```python
from build123d import *

# Parameters (mm, degrees)
PAD_DEPTH       = 51
PAD001_DEPTH    = 22
PAD002_DEPTH    = 66
PAD003_DEPTH    = 1
PAD004_DEPTH    = 25
PAD005_DEPTH    = 51
PAD006_DEPTH    = 17
PAD007_DEPTH    = 17
PAD008_DEPTH    = 17
PAD009_DEPTH    = 41
SKETCH010_W     = 2
SKETCH010_H     = 1
PAD010_DEPTH    = 7
POCKET_DEPTH    = 1
PAD011_DEPTH    = 68
POCKET001_DEPTH = 68
POCKET002_DEPTH = 70
POCKET003_DEPTH = 22
POCKET004_DEPTH = 54
POCKET005_DEPTH = 17
SKETCH018_W     = 3
SKETCH018_H     = 2
POCKET006_DEPTH = 2
POCKET007_DEPTH = 17
PAD012_DEPTH    = 17
PAD013_DEPTH    = 18
POCKET008_DEPTH = 70
SKETCH023_W     = 3
SKETCH023_H     = 5
PAD014_DEPTH    = 103
POCKET009_DEPTH = 13
SKETCH025_W     = 2
SKETCH025_H     = 3
POCKET010_DEPTH = 103
SKETCH026_W     = 3
SKETCH026_H     = 5
PAD015_DEPTH    = 103
SKETCH027_W     = 2
SKETCH027_H     = 3
POCKET011_DEPTH = 103
POCKET012_DEPTH = 31
POCKET013_DEPTH = 45
POCKET014_DEPTH = 28
PAD016_DEPTH    = 44
POCKET015_DEPTH = 51
SKETCH033_W     = 6
SKETCH033_H     = 7
POCKET016_DEPTH = 2


with BuildPart() as part:
    # Sketch → Pad (new body)
    with BuildSketch(Plane.XZ):
        Polygon((0, 0), (15, 0), (15, -2), (14, -3), (1, -3), (0, -2), align=None)
    extrude(amount=PAD_DEPTH)

    # Sketch001 (on Face2 of Pad) → Pad001 (join)
    with BuildSketch(Plane(origin=(5, 0, 0), x_dir=(0, 0, 1), z_dir=(1, 0, 0))):
        Polygon((0, 51), (0, 66), (-2, 66), (-3, 65), (-3, 52), (-2, 51), align=None)
    extrude(amount=PAD001_DEPTH)

    # Sketch002 (on Face14 of Pad001) → Pad002 (join)
    with BuildSketch(Plane(origin=(27, 0, 0), x_dir=(0, 0, 1), z_dir=(1, 0, 0))):
        Polygon((0, 70), (0, 55), (-2, 55), (-3, 56), (-3, 69), (-2, 70), align=None)
    extrude(amount=PAD002_DEPTH)

    # Sketch004 (on Face5 of Pad002) → Pad003 (join)
    with BuildSketch(Plane.XZ.offset(51)):
        Polygon((0, 0), (15, 0), (15, -2), (14, -3), (1, -3), (0, -2), align=None)
    extrude(amount=PAD003_DEPTH)

    # Sketch003 (on Face20 of Pad002) → Pad004 (join)
    with BuildSketch(Plane(origin=(0, -56, 0), x_dir=(1, 0, 0), z_dir=(0, 1, 0))):
        Polygon((93, 0), (78, 0), (78, 2), (79, 3), (92, 3), (93, 2), align=None)
    extrude(amount=PAD004_DEPTH)

    # Sketch005 (on Face38 of Pad004) → Pad005 (join)
    with BuildSketch(Plane(origin=(0, -31, 0), x_dir=(1, 0, 0), z_dir=(0, 1, 0))):
        Polygon((84, 0), (99, 0), (99, 2), (98, 3), (85, 3), (84, 2), align=None)
    extrude(amount=PAD005_DEPTH)

    # Sketch006 (on Face47 of Pad005) → Pad006 (join)
    with BuildSketch(Plane(origin=(0, 13, 0), x_dir=(1, 0, 0), z_dir=(0, 1, 0))):
        Polygon((69, 0), (84, 0), (84, 2), (83, 3), (70, 3), (69, 2), align=None)
    extrude(amount=PAD006_DEPTH)

    # Sketch007 (on Face4 of Pad006) → Pad007 (join)
    with BuildSketch(Plane(origin=(0, 0, 0), x_dir=(1, 0, 0), z_dir=(0, 1, 0))):
        Polygon((8, 0), (23, 0), (23, 2), (22, 3), (9, 3), (8, 2), align=None)
    extrude(amount=PAD007_DEPTH)

    # Sketch008 (on Face17 of Pad007) → Pad008 (join)
    with BuildSketch(Plane(origin=(0, 17, 0), x_dir=(1, 0, 0), z_dir=(0, 1, 0))):
        Polygon((15, 0), (30, 0), (30, 2), (29, 3), (16, 3), (15, 2), align=None)
    extrude(amount=PAD008_DEPTH)

    # Sketch009 (on Face31 of Pad008) → Pad009 (join)
    with BuildSketch(Plane(origin=(29, 0, 0), x_dir=(0, 0, 1), z_dir=(1, 0, 0))):
        Polygon((0, -37), (0, -22), (-2, -22), (-3, -23), (-3, -36), (-2, -37), align=None)
    extrude(amount=PAD009_DEPTH)

    # Sketch010 (on Face81 of Pad009) → Pad010 (join)
    with BuildSketch(Plane(origin=(0, 13, 0), x_dir=(1, 0, 0), z_dir=(0, 1, 0))):
        with Locations((84, 2.5)):
            Rectangle(SKETCH010_W, SKETCH010_H)
    extrude(amount=PAD010_DEPTH)

    # Sketch011 (on Face36 of Pad010) → Pocket (cut)
    with BuildSketch(Plane(origin=(0, 0, 0), x_dir=(-1, 0, 0), z_dir=(0, 0, 1))):
        Polygon((-90.1471723822, 70), (-79, 70), (-90.1471723822, 59.9630409046), align=None)
    extrude(amount=-POCKET_DEPTH, mode=Mode.SUBTRACT)

    # Sketch012 (on Face51 of Pocket) → Pad011 (join)
    with BuildSketch(Plane(origin=(38.0611229336, -42.2711594585, 0), x_dir=(0.7431448255, 0.6691306064, 0), z_dir=(0.6691306064, -0.7431448255, 0))):
        Polygon((11.8692987676, 0), (26.8692987676, 0), (26.8692987676, -2), (25.8692987676, -3), (12.8692987676, -3), (11.8692987676, -2), align=None)
    extrude(amount=PAD011_DEPTH)

    # Sketch013 (on Face80 of Pad011) → Pocket001 (cut)
    with BuildSketch(Plane(origin=(83.562004166, -92.805007591, 0), x_dir=(0.7431448255, 0.6691306064, 0), z_dir=(0.6691306064, -0.7431448255, 0))):
        Polygon((14.8692987676, 0), (23.8692987676, 0), (23.8692987676, -1.5), (24.3692987676, -1.5), (24.3692987676, -2), (14.3692987676, -2), (14.3692987676, -1.5), (14.8692987676, -1.5), align=None)
    extrude(amount=-POCKET001_DEPTH, mode=Mode.SUBTRACT)

    # Sketch014 (on Face46 of Pocket001) → Pocket002 (cut)
    with BuildSketch(Plane(origin=(27, 0, 0), x_dir=(0, 0, -1), z_dir=(-1, 0, 0))):
        Polygon((0, 67), (1.5, 67), (1.5, 67.5), (2, 67.5), (2, 57.5), (1.5, 57.5), (1.5, 58), (0, 58), align=None)
    extrude(amount=-POCKET002_DEPTH, mode=Mode.SUBTRACT)

    # Sketch015 (on Face34 of Pocket002) → Pocket003 (cut)
    with BuildSketch(Plane(origin=(5, 0, 0), x_dir=(0, 0, -1), z_dir=(-1, 0, 0))):
        Polygon((0, 63), (0.5, 63), (0.5, 63.5), (2, 63.5), (2, 53.5), (0.5, 53.5), (0.5, 54), (0, 54), align=None)
    extrude(amount=-POCKET003_DEPTH, mode=Mode.SUBTRACT)

    # Sketch016 (on Face4 of Pocket003) → Pocket004 (cut)
    with BuildSketch(Plane(origin=(0, 0, 0), x_dir=(1, 0, 0), z_dir=(0, 1, 0))):
        Polygon((2.5, 2), (12.5, 2), (12.5, 1.5), (12, 1.5), (12, 0), (3, 0), (3, 1.5), (2.5, 1.5), align=None)
    extrude(amount=-POCKET004_DEPTH, mode=Mode.SUBTRACT)

    # Sketch017 (on Face19 of Pocket004) → Pocket005 (cut)
    with BuildSketch(Plane(origin=(0, 17, 0), x_dir=(1, 0, 0), z_dir=(0, 1, 0))):
        Polygon((11, 0), (11, 1.5), (10.5, 1.5), (10.5, 2), (20.5, 2), (20.5, 1.5), (20, 1.5), (20, 0), align=None)
    extrude(amount=-POCKET005_DEPTH, mode=Mode.SUBTRACT)

    # Sketch018 (on Face48 of Pocket005) → Pocket006 (cut)
    with BuildSketch(Plane(origin=(0, 0, 0), x_dir=(-1, 0, 0), z_dir=(0, 0, 1))):
        with Locations((-11.5, 0)):
            Rectangle(SKETCH018_W, SKETCH018_H)
    extrude(amount=-POCKET006_DEPTH, mode=Mode.SUBTRACT)

    # Sketch019 (on Face63 of Pocket006) → Pocket007 (cut)
    with BuildSketch(Plane(origin=(0, 34, 0), x_dir=(1, 0, 0), z_dir=(0, 1, 0))):
        Polygon((18, 0), (18, 1.5), (17.5, 1.5), (17.5, 2), (27.5, 2), (27.5, 1.5), (27, 1.5), (27, 0), align=None)
    extrude(amount=-POCKET007_DEPTH, mode=Mode.SUBTRACT)

    # Sketch020 (on Face117 of Pocket007) → Pad012 (join)
    with BuildSketch(Plane(origin=(0, 30, 0), x_dir=(1, 0, 0), z_dir=(0, 1, 0))):
        Polygon((70, 3), (83, 3), (84, 2), (84, 0), (69, 0), (69, 2), align=None)
    extrude(amount=PAD012_DEPTH)

    # Sketch021 (on Face108 of Pad012) → Pad013 (join)
    with BuildSketch(Plane.XZ.offset(74.8)):
        Polygon((88.5297845093, 0), (103.5297845093, 0), (103.5297845093, -2), (102.5297845093, -3), (89.5297845093, -3), (88.5297845093, -2), align=None)
    extrude(amount=PAD013_DEPTH)

    # Sketch022 (on Face158 of Pad013) → Pocket008 (cut)
    with BuildSketch(Plane(origin=(38.0611229336, -42.2711594585, 0), x_dir=(0.7431448255, 0.6691306064, 0), z_dir=(-0.6691306064, 0.7431448255, 0))):
        Polygon((14.3692987676, 2), (24.3692987676, 2), (24.3692987676, 1.5), (23.8692987676, 1.5), (23.8692987676, 0), (14.8692987676, 0), (14.8692987676, 1.5), (14.3692987676, 1.5), align=None)
    extrude(amount=-POCKET008_DEPTH, mode=Mode.SUBTRACT)

    # Sketch023 (on Face171 of Pocket008) → Pad014 (join)
    with BuildSketch(Plane(origin=(103.5297845093, 0, 0), x_dir=(0, 0, -1), z_dir=(-1, 0, 0))):
        with Locations((1.5, 90.3)):
            Rectangle(SKETCH023_W, SKETCH023_H)
    extrude(amount=PAD014_DEPTH)

    # Sketch024 (on Face231 of Pad014) → Pocket009 (cut)
    with BuildSketch(Plane.XZ.offset(92.8)):
        Polygon((91.0297845093, -2), (101.0297845093, -2), (101.0297845093, -1.5), (100.5297845093, -1.5), (100.5297845093, 0), (91.5297845093, 0), (91.5297845093, -1.5), (91.0297845093, -1.5), align=None)
    extrude(amount=-POCKET009_DEPTH, mode=Mode.SUBTRACT)

    # Sketch025 (on Face210 of Pocket009) → Pocket010 (cut)
    with BuildSketch(Plane(origin=(0.5297845093, 0, 0), x_dir=(0, 0, -1), z_dir=(-1, 0, 0))):
        with Locations((1, 91.3)):
            Rectangle(SKETCH025_W, SKETCH025_H)
    extrude(amount=-POCKET010_DEPTH, mode=Mode.SUBTRACT)

    # Sketch026 (on Face150 of Pocket010) → Pad015 (join)
    with BuildSketch(Plane(origin=(0.5, 0, 0), x_dir=(0, 0, 1), z_dir=(1, 0, 0))):
        with Locations((-1.5, -44.5)):
            Rectangle(SKETCH026_W, SKETCH026_H)
    extrude(amount=PAD015_DEPTH)

    # Sketch027 (on Face187 of Pad015) → Pocket011 (cut)
    with BuildSketch(Plane(origin=(103.5, 0, 0), x_dir=(0, 0, 1), z_dir=(1, 0, 0))):
        with Locations((-1, -45.5)):
            Rectangle(SKETCH027_W, SKETCH027_H)
    extrude(amount=-POCKET011_DEPTH, mode=Mode.SUBTRACT)

    # Sketch028 (on Face117 of Pocket011) → Pocket012 (cut)
    with BuildSketch(Plane.XZ.offset(-13)):
        Polygon((71.5, -2), (81.5, -2), (81.5, -1.5), (81, -1.5), (81, 0), (72, 0), (72, -1.5), (71.5, -1.5), align=None)
    extrude(amount=-POCKET012_DEPTH, mode=Mode.SUBTRACT)

    # Sketch029 (on Face87 of Pocket012) → Pocket013 (cut)
    with BuildSketch(Plane(origin=(27, 0, 0), x_dir=(0, 0, -1), z_dir=(-1, 0, 0))):
        Polygon((2, -24.5), (2, -34.5), (1.5, -34.5), (1.5, -34), (0, -34), (0, -25), (1.5, -25), (1.5, -24.5), align=None)
    extrude(amount=-POCKET013_DEPTH, mode=Mode.SUBTRACT)

    # Sketch030 (on Face210 of Pocket013) → Pocket014 (cut)
    with BuildSketch(Plane(origin=(0, -31, 0), x_dir=(1, 0, 0), z_dir=(0, 1, 0))):
        Polygon((80.5, 2), (90.5, 2), (90.5, 1.5), (90, 1.5), (90, 0), (81, 0), (81, 1.5), (80.5, 1.5), align=None)
    extrude(amount=-POCKET014_DEPTH, mode=Mode.SUBTRACT)

    # Sketch031 (on Face234 of Pocket014) → Pad016 (join)
    with BuildSketch(Plane(origin=(0, -31, 0), x_dir=(1, 0, 0), z_dir=(0, 1, 0))):
        Polygon((78, 2), (79, 3), (85, 3), (85, 2), (80.5, 2), (80.5, 1.5), (81, 1.5), (81, 0), (78, 0), align=None)
    extrude(amount=PAD016_DEPTH)

    # Sketch032 (on Face205 of Pad016) → Pocket015 (cut)
    with BuildSketch(Plane(origin=(0, 20, 0), x_dir=(1, 0, 0), z_dir=(0, 1, 0))):
        Polygon((86.5, 2), (96.5, 2), (96.5, 1.5), (96, 1.5), (96, 0), (87, 0), (87, 1.5), (86.5, 1.5), align=None)
    extrude(amount=-POCKET015_DEPTH, mode=Mode.SUBTRACT)

    # Sketch033 (on Face207 of Pocket015) → Pocket016 (cut)
    with BuildSketch(Plane(origin=(0, 0, 0), x_dir=(-1, 0, 0), z_dir=(0, 0, 1))):
        with Locations((-84, -16.5)):
            Rectangle(SKETCH033_W, SKETCH033_H)
    extrude(amount=-POCKET016_DEPTH, mode=Mode.SUBTRACT)


solid = part.part
```
For this review, take the finished solid that the model builds, in its own axes (mm). A direction names the side the tool comes from. Round coordinates to 2 decimals unless told otherwise and drop trailing zeros. Write each loop counter-clockwise with the first axis right and the second up, starting at its lowest first coordinate (ties: lowest second). Pieces come first, ordered by that corner, then holes. Notation, with made-up numbers: M 23.25,-25.75 L 46.25,-25.75 A22 ccw 46.25,7.25 Z; hole C 82.25,26.5 d7. An arc over 180 degrees is marked long. One line per item, written item: value. Start each with the question number.
(1) Machinability: for faces 1 (the flat face through (43.7, 42.4, 0)), 2 (the flat face through (20.3, 34, -2.2)), 3 (the flat face through (98.224, -72.669, -1.754)), 4 (the flat face through (67.875, -35.227, -0.986)), which of the approach directions +Z, -Z, +X, -X, +Y, -Y give a long, thin tool a straight path to every point of the face, cutting with its end or side? Answer none if there is none.
(2) Insertion check: pin 1 (1.2 mm diameter, centred on y = -14.5, z = -1, fed in from +X); pin 2 (0.8 mm diameter, centred on y = 9, z = -0.5, fed in from -X); pin 3 (0.9 mm diameter, centred on y = -44, z = -2, fed in from +X); pin 4 (10 mm diameter, centred on x = 50.5, y = -18, fed in from +Z). Each pin has a flat end and moves straight along its axis. Give the tip position at first contact, or say it passes through.
(3) We need section C-C (x = 42). Count the separate pieces of the cut face and the enclosed holes in it, and give its area (3 significant figures).
(4) Wall thickness on line 1 (X direction, y = -21.5, z = -1.8); line 2 (Y direction, x = 17, z = -1); line 3 (X direction, y = -10.5, z = -0.3): over which ranges is each line inside the solid? List them lowest first.
(5) The part is to be moulded in two halves that separate along Y. For faces 5 (the flat face through (96.5, -71, -1.5)), 6 (the flat face through (5, -60.7, -2.2)), 7 (the flat face through (97, -5, 0)), say which applies: released by +Y, released by -Y, zero draft, split by the parting line, or undercut.
(6) We need section B-B (y = -83). Give the boundary of the cut face in (x, z), and give its area (3 significant figures).
Result:
1. face 1: +Z, +X, -X, +Y, -Y
1. face 2: +Z, -Z, -X
1. face 3: none
1. face 4: +Z, -Z
2. pin 1: x = 99
2. pin 2: x = 8
2. pin 3: x = 93
2. pin 4: through
3. separate pieces: 4
3. enclosed holes: 0
3. area: 69.0 mm²
4. line 1: 0 to 2.5, 12.5 to 15, 78 to 80.5, 84 to 86.5, 96.5 to 99
4. line 2: -89.8 to -87.8, -66 to -63.5, -53.5 to -51, 17 to 34, 42 to 44
4. line 3: 0 to 3, 12 to 15, 78 to 81, 84 to 87, 96 to 99
5. face 5: undercut
5. face 6: undercut
5. face 7: zero draft
6. outline: M 88.53,-2 L 89.53,-3 L 102.53,-3 L 103.53,-2 L 103.53,0 L 100.53,0 L 100.53,-1.5 L 101.03,-1.5 L 101.03,-2 L 91.03,-2 L 91.03,-1.5 L 91.53,-1.5 L 91.53,0 L 88.53,0 Z
6. area: 25.5 mm²
